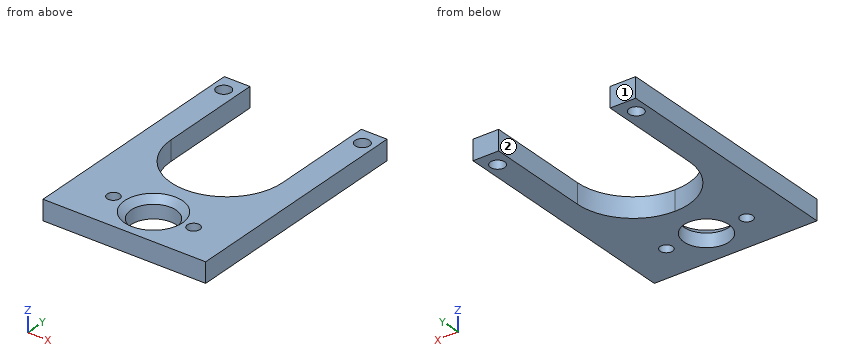
from build123d import *

# Parameters (mm, degrees)
ESQUISSE1_R             = 7.14375
ESQUISSE1_R_2           = 2.286
BOSS_EXTRU_1_DEPTH      = 6.35
ESQUISSE3_R             = 1.984375
ENL_V_MAT_EXTRU_1_DEPTH = 70.699220992
BOSS_EXTRUDE1_DEPTH     = 6.35
CHAMFER1_SIZE           = 2.032


with BuildPart() as part:
    # Esquisse1 → Boss.-Extru.1 (new body)
    with BuildSketch(Plane.XY):
        Polygon((-26.06959879, 64.327559614), (-17.94159879, 64.327559614), (-17.94159879, 13.527559614), (17.36440121, 13.527559614), (17.36440121, 64.327559614), (25.49240121, 64.327559614), (25.49240121, -11.872440386), (-26.06959879, -11.872440386), align=None)
        Circle(ESQUISSE1_R, mode=Mode.SUBTRACT)
        with Locations((21.68240121, 59.024929956)):
            Circle(ESQUISSE1_R_2, mode=Mode.SUBTRACT)
        with Locations((-22.25959879, 59.024929956)):
            Circle(ESQUISSE1_R_2, mode=Mode.SUBTRACT)
    extrude(amount=BOSS_EXTRU_1_DEPTH)

    # Esquisse3 → Enlèv. mat.-Extru.1 (cut, through all)
    with BuildSketch(Plane.XY.offset(6.35)):
        with Locations((12.7, 0)):
            Circle(ESQUISSE3_R)
    enl_v_mat_extru_1 = extrude(amount=-ENL_V_MAT_EXTRU_1_DEPTH, mode=Mode.SUBTRACT)

    # Symétrie1: Enlèv. mat.-Extru.1 across plane
    add(enl_v_mat_extru_1.mirror(Plane(origin=(0, 0, 0), x_dir=(0, 0, 1), z_dir=(1, 0, 0))), mode=Mode.SUBTRACT)

    # Sketch1 → Boss-Extrude1 (add)
    with BuildSketch(Plane.XY.offset(6.35)):
        with BuildLine():
            ThreePointArc((-0.28859879, 13.527559614), (-12.771154798, 18.698003606), (-17.94159879, 31.180559614))
            Line((-17.94159879, 31.180559614), (-17.94159879, 13.527559614))
            Line((-17.94159879, 13.527559614), (-0.28859879, 13.527559614))
        make_face()
        with BuildLine():
            ThreePointArc((17.36440121, 31.180559614), (12.193957219, 18.698003606), (-0.28859879, 13.527559614))
            Line((-0.28859879, 13.527559614), (17.36440121, 13.527559614))
            Line((17.36440121, 13.527559614), (17.36440121, 31.180559614))
        make_face()
    extrude(amount=-BOSS_EXTRUDE1_DEPTH)

    # Chamfer1
    chamfer1_edges = [part.edges().sort_by_distance(p)[0] for p in [
        (-7.14375, 0, 6.35),
    ]]
    chamfer(chamfer1_edges, length=CHAMFER1_SIZE)


solid = part.part
Input: part model. Units: mm. Frame: model coordinates. Face numbers are marked on the shaded views. A direction names the side the tool comes from. Round coordinates to 2 decimals unless told otherwise and drop trailing zeros. Loops run counter-clockwise (first coordinate to the right, second up) from the corner with the lowest first, then second, coordinate; pieces in that order, holes last. Notation, with made-up numbers: (-0.75, -16.5) -> (28.25, -16.5) arc R23 cw to (28.25, 5.5) -> close; hole circle Ø1 at (45.5, 10.25). An arc over 180 degrees is marked (long way). Answer as a JSON object with one key per item and string values. Group by question number.
1) Reachability of the marked faces 1 and 2 from +Z, -Z, +X, -X, +Y, -Y: full face, straight path, thin tool, end or side. Return the list, or none.
2) Section query A-A on y = 0. Output: boundary loops of the cut face in (x, z).
3) Section query C-C on z = 2.5. Output: boundary loops of the cut face in (x, y), plus the area to 3 significant figures.
4) Section query B-B on x = -13. Output: boundary loops of the cut face in (y, z).
5) Ray query, L1, parallel to Y at x = 0, z = 2.9; L2, parallel to X at y = 46.5, z = 4.5; L3, parallel to X at y = 1.5, z = 2.25. Return the intervals inside material, ascending.
6) Section query D-D on y = 28.5. Output: boundary loops of the cut face in (x, z).
Reply:
{
 "1": {"face 1": "+Z, -Z, +X, -X, +Y", "face 2": "+Z, -Z, +Y"},
 "2": {"outline": "(-26.07, 0) -> (-14.68, 0) -> (-14.68, 6.35) -> (-26.07, 6.35) -> close; (-10.72, 0) -> (-7.14, 0) -> (-7.14, 4.32) -> (-9.18, 6.35) -> (-10.72, 6.35) -> close; (7.14, 0) -> (10.72, 0) -> (10.72, 6.35) -> (9.18, 6.35) -> (7.14, 4.32) -> close; (14.68, 0) -> (25.49, 0) -> (25.49, 6.35) -> (14.68, 6.35) -> close"},
 "3": {"outline": "(-26.07, -11.87) -> (25.49, -11.87) -> (25.49, 64.33) -> (17.36, 64.33) -> (17.36, 31.18) arc R17.65 cw to (-17.94, 31.18) -> (-17.94, 64.33) -> (-26.07, 64.33) -> close; hole circle Ø4.57 at (-22.26, 59.02); hole circle Ø3.97 at (-12.7, 0); hole circle Ø14.29 at (0, 0); hole circle Ø3.97 at (12.7, 0); hole circle Ø4.57 at (21.68, 59.02)", "area": "2,050 mm2"},
 "4": {"outline": "(-11.87, 0) -> (-1.96, 0) -> (-1.96, 6.35) -> (-11.87, 6.35) -> close; (1.96, 0) -> (18.93, 0) -> (18.93, 6.35) -> (1.96, 6.35) -> close"},
 "5": {"L1": "y = -11.87 to -7.14, 7.14 to 13.53", "L2": "x = -26.07 to -17.94, 17.36 to 25.49", "L3": "x = -26.07 to -14, -11.4 to -6.98, 6.98 to 11.4, 14 to 25.49"},
 "6": {"outline": "(-26.07, 0) -> (-17.74, 0) -> (-17.74, 6.35) -> (-26.07, 6.35) -> close; (17.16, 0) -> (25.49, 0) -> (25.49, 6.35) -> (17.16, 6.35) -> close"}
}
